Could you check a few things on this model? Use its own coordinates, in mm. A direction names the side the tool comes from. Give positions to 0.01 mm unless a question says otherwise; leave off trailing zeros. Write each loop counter-clockwise with the first axis right and the second up, starting at its lowest first coordinate (ties: lowest second). Pieces come first, ordered by that corner, then holes. Notation, with made-up numbers: (18, -7.5) - (41, -7.5) arc R14 cw to (41, 19.5) - close; hole circle Ø9 at (-17, 77.5). An arc over 180 degrees is marked (long way). Use one line per item in the form item = value.
Solid Edge part; units mm, degrees
sketch "Sketch1" plane through (0, 0, 0) normal (0, -1, 0) x (1, 0, 0)
  circle A0 centre (0, 0) radius 40.4368
  circle A1 centre (0, 0) radius 50.8
extrude "Protrusion1" add sketch "Sketch1" along normal blind 8.89
sketch "Sketch2" plane through (0, 0, 0) normal (0, 0, 1) x (1, 0, 0)
  line L0 (44.2468, 5.08) -> (40.4368, 0)
  line L1 (40.4368, 0) -> (48.0568, 0)
  line L2 (44.2468, 5.08) -> (48.0568, 0)
revolve "RevolvedProtrusion1" add sketch "Sketch2" angle 360 about axis through (0, 0, 0) along (0, 1, 0)
sketch "Sketch3" plane through (0, 0, 0) normal (0, 1, 0) x (-1, 0, 0)
  circle A0 centre (0, 49.4284) radius 0.9525
extrude "Cutout1" cut sketch "Sketch3" against normal through all
pattern_circular "Pattern_2" count 16 over 360 about axis through (0, 0, 0) along (0, 1, 0) of "Cutout1"
sketch "Sketch4" plane through (0, 0, 0) normal (0, -1, 0) x (1, 0, 0)
  circle A0 centre (0, 0) radius 57.15
  circle A1 centre (0, 0) radius 50.8
extrude "Protrusion2" add sketch "Sketch4" along normal up to vertex (8.89 mm away)
sketch "Sketch5" plane through (0, 0, 0) normal (0, 1, 0) x (-1, 0, 0)
  line L0 (-57.15, 0) -> (-50.8, 0)
  line L1 (50.8, 0) -> (57.15, 0)
  arc A0 (50.8, 0) -> (-50.8, 0) centre (0, 0) cw
  arc A1 (57.15, 0) -> (-57.15, 0) centre (0, 0) cw
extrude "ExtrudedCutout_34" cut sketch "Sketch5" against normal blind 6.35
fillet "Round_1" radius 6.35 2 edges at (53.975, -6.35, 0) (-53.975, -6.35, 0)
1. Imagine slicing it at B-B, the plane y = 2.5. List the corners of the cut face in (x, z) for me, and give its area (3 significant figures).
Response values:
outline = circle Ø92.36 at (0, 0); hole circle Ø84.62 at (0, 0)
area = 1,080 mm²
2. Which directions (+Z, -Z, +X, -X, +Y, -Y) give clear straight access to the entire face, cutting with the end or side of a thin tool? Please do faces 1 (the face through (-12, -8.89, 39)), 2 (the face through (-53.73, -4.44, -1.81)), 3 (the face through (1.117, -3.131, -50.788)), 4 (the face through (-12, 0, 47)), 5 (the face through (-8.766, -4.383, 39.475)).
Response values:
face_1 = +Z, -Z, +X, -X, -Y
face_2 = -Z, -X, +Y
face_3 = -Z, +Y
face_4 = +Y
face_5 = +Y, -Y
3. If we mould it in two halves opening along X, with no side actions, what happens to faces 6 (the face through (53.82, -4.44, -1.81)), 7 (the face through (-12.39, -5.37, 55.79)), 8 (the face through (-8.8, 0.3, 39.7))? For each: pulls with the +X half, pulls with the -X half, needs draft (parallel to the pull), parting line crosses it, or undercut.
Response values:
face_6 = needs draft
face_7 = parting line crosses it
face_8 = undercut
4. Imagine slicing it at A-A, the plane y = -4. State how many separate pieces and enclosed holes the cut face has, and give its area (3 significant figures).
Response values:
separate_pieces = 1
enclosed_holes = 17
area = 4,020 mm²
5. If I drill on line 1 (Z direction, x = 0, y = -7); line 2 (Z direction, x = 0, y = -5.75); line 3 (X direction, y = -4.5, z = -45.5), over which ranges is the centre line in solid material (lowest first)? Write a range as from..to.
Response values:
line_1 = -57.15..-50.38, -48.48..-40.44, 40.44..48.48, 50.38..57.15
line_2 = -50.8..-50.38, -48.48..-40.44, 40.44..48.48, 50.38..57.15
line_3 = -22.59..-19.85, -17.98..17.98, 19.85..22.59
6. For pin 1 (2 mm diameter, centred on x = -18.92, z = 45.67, fed in from +Y); pin 2 (5 mm diameter, centred on y = -6.5, z = -30.5, fed in from -X); pin 3 (15 mm diameter, centred on x = -23.5, z = -21.5, fed in from +Y); pin 4 (1 mm diameter, centred on y = -1, z = -43.5, fed in from +X), each with a flat end and sliding along its axis, tell me the tip position at first contact or that it passes through.
Response values:
pin_1 = 0
pin_2 = -49.82
pin_3 = through
pin_4 = 27.05
